For this review, take the finished solid that the model builds, in its own axes (mm). Coordinates: 2 decimals unless noted, no trailing zeros. Write each loop counter-clockwise with the first axis right and the second up, starting at its lowest first coordinate (ties: lowest second). Pieces come first, ordered by that corner, then holes. Notation, with made-up numbers: (56.5, 50) -> (67.5, 50) arc R13 cw to (67.5, 66) -> close; hole circle Ø11 at (4, -12.5). An arc over 180 degrees is marked (long way). Put each result on its own line as item: value. Start each with the question number.
Item 1: Consider section B-B on x = -10. Give the boundary of the cut face in (y, z).
Item 2: Consider section A-A on y = 0. Give the boundary of the cut face in (x, z), and give its area (3 significant figures).
Item 3: To check wall thickness, follow L1, parallel to X at y = 2, z = 0; L2, parallel to Y at x = 0, z = -8; L3, parallel to Z at x = 10, y = -1.75. State the ranges of each line that lie inside material, in increasing order.
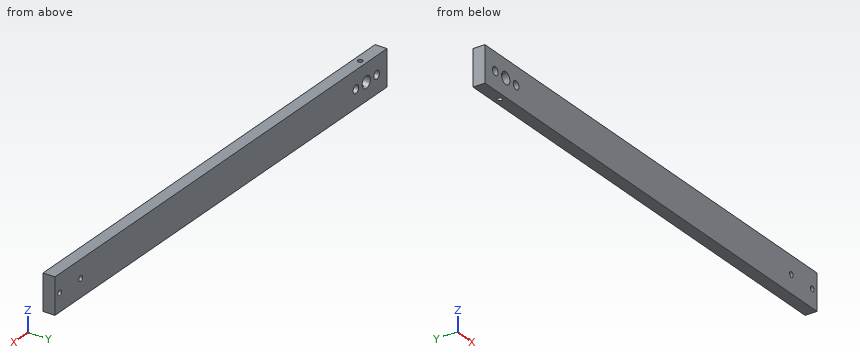
```python
from build123d import *

# Parameters (mm, degrees)
BOSS_EXTRUDE1_DEPTH              = 4
BOSS_EXTRUDE1_DEPTH_BACK         = 4
SKETCH1_W                        = 320
SKETCH1_H                        = 24
SKETCH1_R                        = 2.75
SKETCH1_R_2                      = 1.75
SKETCH1_R_3                      = 4
TAP_DRILL_FOR_M4X0_7_TAP1_REACH  = 302.985
TAP_DRILL_FOR_M4X0_7_TAP1_BORE_R = 1.65
TAP_DRILL_FOR_M4X0_7_TAP2_D      = 3.3


with BuildPart() as part:
    # Sketch1 → Boss-Extrude1 (new, two sides: drawn at the far end of the back side and taken through both)
    with BuildSketch(Plane(origin=(0, 0, 0), x_dir=(1, 0, 0), z_dir=(0, 1, 0)).offset(-BOSS_EXTRUDE1_DEPTH_BACK)):
        with Locations((140, 0)):
            Rectangle(SKETCH1_W, SKETCH1_H)
        with Locations(Location((-10, 0, 0), (0, 0, 270))):
            Circle(SKETCH1_R, mode=Mode.SUBTRACT)
        with Locations(Location((10, 0, 0), (0, 0, 90))):
            Circle(SKETCH1_R, mode=Mode.SUBTRACT)
        with Locations(Location((295.5, 0, 0), (0, 0, 270))):
            Circle(SKETCH1_R_2, mode=Mode.SUBTRACT)
        with Locations(Location((275.3, 0, 0), (0, 0, 270))):
            Circle(SKETCH1_R_2, mode=Mode.SUBTRACT)
        with Locations(Location((0, 0, 0), (0, 0, 270))):
            Circle(SKETCH1_R_3, mode=Mode.SUBTRACT)
    extrude(amount=BOSS_EXTRUDE1_DEPTH + BOSS_EXTRUDE1_DEPTH_BACK)

    # Tap Drill for M4x0.7 Tap1 bore → Tap Drill for M4x0.7 Tap1 (cut, up to next)
    with BuildSketch(Plane.XY.offset(12), mode=Mode.PRIVATE) as tap_drill_for_m4x0_7_tap1_sk1:
        Circle(TAP_DRILL_FOR_M4X0_7_TAP1_BORE_R)
    tap_drill_for_m4x0_7_tap1_tool1 = extrude(tap_drill_for_m4x0_7_tap1_sk1.sketch, amount=-TAP_DRILL_FOR_M4X0_7_TAP1_REACH, mode=Mode.PRIVATE) & part.part
    add(tap_drill_for_m4x0_7_tap1_tool1.solids().sort_by_distance((0, 0, 12))[0], mode=Mode.SUBTRACT)

    # Tap Drill for M4x0.7 Tap2 (through all)
    with Locations(Plane(origin=(0, 0, -12), x_dir=(-1, 0, 0), z_dir=(0, 0, -1))):
        with Locations((0, 0)):
            Hole(TAP_DRILL_FOR_M4X0_7_TAP2_D / 2)


solid = part.part
```
Return value:
1. outline: (-4, -12) -> (4, -12) -> (4, -2.75) -> (-4, -2.75) -> close; (-4, 2.75) -> (4, 2.75) -> (4, 12) -> (-4, 12) -> close
2. outline: (-20, -12) -> (-1.65, -12) -> (-1.65, -3.64) arc R4 cw to (-1.65, 3.64) -> (-1.65, 12) -> (-20, 12) -> close; (1.65, -12) -> (300, -12) -> (300, 12) -> (1.65, 12) -> (1.65, 3.64) arc R4 cw to (1.65, -3.64) -> close; hole circle Ø5.5 at (-10, 0); hole circle Ø5.5 at (10, 0); hole circle Ø3.5 at (275.3, 0); hole circle Ø3.5 at (295.5, 0)
2. area: 7,510 mm^2
3. L1: -20 to -12.75, -7.25 to -4, 4 to 7.25, 12.75 to 273.55, 277.05 to 293.75, 297.25 to 300
3. L2: -4 to -1.65, 1.65 to 4
3. L3: -12 to -2.75, 2.75 to 12
